The model under review builds one solid part; all positions refer to its coordinate system, in mm. Face numbers are marked on the shaded views. A direction names the side the tool comes from. Round coordinates to 2 decimals unless told otherwise and drop trailing zeros. Order: outer loops, then holes, each group sorted by start corner. A loop starts at its lowest first (then second) coordinate and runs counter-clockwise, first axis right, second up.
1) Machinability: for the marked faces 1 and 2, which of the approach directions +Z, -Z, +X, -X, +Y, -Y give a long, thin tool a straight path to every point of the face, cutting with its end or side? Answer none if there is none.
2) Consider section B-B (y = 5). Give the boundary of the cut face in (x, z) (3 decimals).
3) Mouldability with a two-part tool opening along Z and no side actions: class the marked faces 3 and 4 as pulls with the +Z half, pulls with the -Z half, needs draft (parallel to the pull), parting line crosses it, or undercut.
4) Consider section C-C (z = -12.5). Give the boundary of the cut face in (x, y), then the cut area to 3 significant figures.
5) Consider section A-A (z = -36). Give the boundary of the cut face in (x, y) (3 decimals), then the cut area to 3 significant figures.
6) Clearance check with flat-ended pins moving along their axes: P1, Ø0.6, axis at y = 0.5, z = -29.5, coming from the +X side (3 decimals); P2, Ø1.2, axis at x = 0, z = -36, coming from the +Y side; P3, Ø1.6, axis at y = 1, z = -8.5, coming from the +X side; P4, Ø2, axis at x = 26.5, y = 5, coming from the -Z side. State where each tip first meets the part, or that it passes through.
7) To check wall thickness, follow L1, parallel to X at y = 2.8, z = -7.5 (3 decimals); L2, parallel to Z at x = -12, y = 3.5; L3, parallel to X at y = 1.25, z = -6.5. State the ranges of each line that lie inside material, in increasing order.
from build123d import *

# Parameters (mm, degrees)
SALIENTE_EXTRUIR1_DEPTH = 4
SALIENTE_EXTRUIR2_START = 4
SALIENTE_EXTRUIR2_DEPTH = 4
REDONDEO1_R             = 10
REDONDEO3_R             = 2
CROQUIS3_R              = 1
CROQUIS3_R_2            = 9
CORTAR_EXTRUIR1_DEPTH   = 2
CROQUIS3_3_R            = 1
CORTAR_EXTRUIR2_DEPTH   = 77.740023923


with BuildPart() as part:
    # Croquis1 → Saliente-Extruir1 (new body)
    with BuildSketch(Plane(origin=(0, 0, 0), x_dir=(1, 0, 0), z_dir=(0, 1, 0))):
        with BuildLine():
            Line((30.125, 7.5), (25.125, 7.5))
            Line((25.125, 7.5), (25.125, 48))
            Line((25.125, 48), (30.125, 48))
            ThreePointArc((30.125, 48), (23.644737534, 63.644737534), (8, 70.125))
            Line((8, 70.125), (8, 65.125))
            Line((8, 65.125), (-8, 65.125))
            Line((-8, 65.125), (-8, 70.125))
            ThreePointArc((-8, 70.125), (-23.644737534, 63.644737534), (-30.125, 48))
            Line((-30.125, 48), (-25.125, 48))
            Line((-25.125, 48), (-25.125, 7.5))
            Line((-25.125, 7.5), (-30.125, 7.5))
            ThreePointArc((-30.125, 7.5), (-26.427223112, -1.427223112), (-17.5, -5.125))
            Line((-17.5, -5.125), (-17.5, -0.125))
            Line((-17.5, -0.125), (17.5, -0.125))
            Line((17.5, -0.125), (17.5, -5.125))
            ThreePointArc((17.5, -5.125), (26.427223112, -1.427223112), (30.125, 7.5))
        make_face()
    extrude(amount=SALIENTE_EXTRUIR1_DEPTH)

    # Croquis1<3> → Saliente-Extruir2 (add)
    with BuildSketch(Plane(origin=(0, 0, 0), x_dir=(1, 0, 0), z_dir=(0, 1, 0)).offset(SALIENTE_EXTRUIR2_START)):
        with BuildLine():
            Line((-30.125, 48), (-25.125, 48))
            ThreePointArc((-25.125, 48), (-20.109203628, 60.109203628), (-8, 65.125))
            Line((-8, 65.125), (-8, 70.125))
            ThreePointArc((-8, 70.125), (-23.644737534, 63.644737534), (-30.125, 48))
        make_face()
        with BuildLine():
            Line((-17.5, -5.125), (-17.5, -0.125))
            ThreePointArc((-17.5, -0.125), (-22.891689207, 2.108310793), (-25.125, 7.5))
            Line((-25.125, 7.5), (-30.125, 7.5))
            ThreePointArc((-30.125, 7.5), (-26.427223112, -1.427223112), (-17.5, -5.125))
        make_face()
        with BuildLine():
            ThreePointArc((25.125, 7.5), (22.891689207, 2.108310793), (17.5, -0.125))
            Line((17.5, -0.125), (17.5, -5.125))
            ThreePointArc((17.5, -5.125), (26.427223112, -1.427223112), (30.125, 7.5))
            Line((30.125, 7.5), (25.125, 7.5))
        make_face()
        with BuildLine():
            ThreePointArc((8, 65.125), (20.109203628, 60.109203628), (25.125, 48))
            Line((25.125, 48), (30.125, 48))
            ThreePointArc((30.125, 48), (23.644737534, 63.644737534), (8, 70.125))
            Line((8, 70.125), (8, 65.125))
        make_face()
    extrude(amount=SALIENTE_EXTRUIR2_DEPTH)

    # Redondeo1
    # the kernel refuses this fillet: 10 mm, written as the material it adds along each edge
    with BuildSketch(Plane(origin=(8, 0, -65.125), x_dir=(-1, 0, 0), z_dir=(0, 1, 0)), Plane(origin=(-17.5, 0, 0.125), x_dir=(1, 0, 0), z_dir=(0, 1, 0)), Plane(origin=(-25.125, 0, -48), x_dir=(0, 0, 1), z_dir=(0, 1, 0))) as redondeo1_piece_1:
        with BuildLine():
            CenterArc((8.660254038, -10), REDONDEO1_R, 90, 60)
            Line((0, -5), (-0.173205081, -4.9))
            ThreePointArc((-0.173205081, -4.9), (-0.2, -2.5), (-0.2, 0))
            Line((-0.2, 0), (0, 0.2))
            Line((0, 0.2), (8.660254038, 0.2))
            Line((8.660254038, 0.2), (8.660254038, 0))
        make_face()
    extrude(amount=4)
    with BuildSketch(Plane(origin=(-8, 0, -65.125), x_dir=(0, 0, -1), z_dir=(0, 1, 0)), Plane(origin=(17.5, 0, 0.125), x_dir=(0, 0, 1), z_dir=(0, 1, 0)), Plane(origin=(25.125, 0, -48), x_dir=(1, 0, 0), z_dir=(0, 1, 0)), Plane(origin=(-25.125, 0, -7.5), x_dir=(-1, 0, 0), z_dir=(0, 1, 0))) as redondeo1_piece_2:
        with BuildLine():
            CenterArc((10, -8.660254038), REDONDEO1_R, 120, 60)
            Line((0, -8.660254038), (-0.2, -8.660254038))
            Line((-0.2, -8.660254038), (-0.2, 0))
            Line((-0.2, 0), (0, 0.2))
            ThreePointArc((0, 0.2), (2.5, 0.2), (4.9, 0.173205081))
            Line((4.9, 0.173205081), (5, 0))
        make_face()
    extrude(amount=4)
    with BuildSketch(Plane(origin=(25.125, 0, -7.5), x_dir=(1, 0, 0), z_dir=(0, 1, 0))) as redondeo1_piece_3:
        with BuildLine():
            CenterArc((10, 8.660254038), REDONDEO1_R, 180, 60)
            Line((0, 8.660254038), (-0.2, 8.660254038))
            Line((-0.2, 8.660254038), (-0.2, 0))
            Line((-0.2, 0), (0, -0.2))
            ThreePointArc((0, -0.2), (2.5, -0.2), (4.9, -0.173205081))
            Line((4.9, -0.173205081), (5, 0))
        make_face()
    extrude(amount=4)

    # Redondeo3
    redondeo3_edges = [part.edges().sort_by_distance(p)[0] for p in [
        (-23.644737534, 8, -63.644737534),
        (-26.427223112, 8, 1.427223112),
        (26.427223112, 8, 1.427223112),
        (23.644737534, 8, -63.644737534),
    ]]
    fillet(redondeo3_edges, radius=REDONDEO3_R)

    # Croquis3 → Cortar-Extruir1 (cut)
    # profile 1 of 5: a face of its own
    with BuildSketch(Plane(origin=(0, 0, 0), x_dir=(1, 0, 0), z_dir=(0, 1, 0))):
        with BuildLine():
            ThreePointArc((-9.5, 10.354191767), (-3, 19), (-9.5, 27.645808233))
            Line((-9.5, 27.645808233), (-9.5, 31.845808233))
            ThreePointArc((-9.5, 31.845808233), (-10.144365081, 33.401443152), (-11.7, 34.045808233))
            Line((-11.7, 34.045808233), (-12.3, 34.045808233))
            ThreePointArc((-12.3, 34.045808233), (-13.855634919, 33.401443152), (-14.5, 31.845808233))
            Line((-14.5, 31.845808233), (-14.5, 27.645808233))
            ThreePointArc((-14.5, 27.645808233), (-21, 19), (-14.5, 10.354191767))
            Line((-14.5, 10.354191767), (-14.5, 6.154191767))
            ThreePointArc((-14.5, 6.154191767), (-13.855634919, 4.598556848), (-12.3, 3.954191767))
            Line((-12.3, 3.954191767), (-11.7, 3.954191767))
            ThreePointArc((-11.7, 3.954191767), (-10.144365081, 4.598556848), (-9.5, 6.154191767))
            Line((-9.5, 6.154191767), (-9.5, 10.354191767))
        make_face()
        with Locations(Location((-12, 7.5, 0), (0, 0, 90))):
            Circle(CROQUIS3_R, mode=Mode.SUBTRACT)
        with Locations(Location((-12, 30.5, 0), (0, 0, 90))):
            Circle(CROQUIS3_R, mode=Mode.SUBTRACT)
    # profile 2 of 5: a face of its own
    with BuildSketch(Plane(origin=(0, 0, 0), x_dir=(1, 0, 0), z_dir=(0, 1, 0))):
        with BuildLine():
            Line((14.5, 27.645808233), (14.5, 31.845808233))
            ThreePointArc((14.5, 31.845808233), (13.855634919, 33.401443152), (12.3, 34.045808233))
            Line((12.3, 34.045808233), (11.7, 34.045808233))
            ThreePointArc((11.7, 34.045808233), (10.144365081, 33.401443152), (9.5, 31.845808233))
            Line((9.5, 31.845808233), (9.5, 27.645808233))
            ThreePointArc((9.5, 27.645808233), (3, 19), (9.5, 10.354191767))
            Line((9.5, 10.354191767), (9.5, 6.154191767))
            ThreePointArc((9.5, 6.154191767), (10.144365081, 4.598556848), (11.7, 3.954191767))
            Line((11.7, 3.954191767), (12.3, 3.954191767))
            ThreePointArc((12.3, 3.954191767), (13.855634919, 4.598556848), (14.5, 6.154191767))
            Line((14.5, 6.154191767), (14.5, 10.354191767))
            ThreePointArc((14.5, 10.354191767), (21, 19), (14.5, 27.645808233))
        make_face()
        with Locations(Location((12, 7.5, 0), (0, 0, 90))):
            Circle(CROQUIS3_R, mode=Mode.SUBTRACT)
        with Locations(Location((12, 30.5, 0), (0, 0, 90))):
            Circle(CROQUIS3_R, mode=Mode.SUBTRACT)
    # profile 3 of 5: a face of its own
    with BuildSketch(Plane(origin=(0, 0, 0), x_dir=(1, 0, 0), z_dir=(0, 1, 0))):
        with Locations((0, 47.5)):
            Circle(CROQUIS3_R_2)
    # profile 4 of 5: a face of its own
    with BuildSketch(Plane(origin=(0, 0, 0), x_dir=(1, 0, 0), z_dir=(0, 1, 0))):
        with BuildLine():
            Line((2.5, 34.654191767), (2.5, 38.854191767))
            ThreePointArc((2.5, 38.854191767), (0, 38.5), (-2.5, 38.854191767))
            Line((-2.5, 38.854191767), (-2.5, 34.654191767))
            ThreePointArc((-2.5, 34.654191767), (-1.855634919, 33.098556848), (-0.3, 32.454191767))
            Line((-0.3, 32.454191767), (0.3, 32.454191767))
            ThreePointArc((0.3, 32.454191767), (1.855634919, 33.098556848), (2.5, 34.654191767))
        make_face()
        with Locations(Location((0, 36, 0), (0, 0, 90))):
            Circle(CROQUIS3_R, mode=Mode.SUBTRACT)
    # profile 5 of 5: a face of its own
    with BuildSketch(Plane(origin=(0, 0, 0), x_dir=(1, 0, 0), z_dir=(0, 1, 0))):
        with BuildLine():
            ThreePointArc((-2.5, 56.145808233), (0, 56.5), (2.5, 56.145808233))
            Line((2.5, 56.145808233), (2.5, 60.345808233))
            ThreePointArc((2.5, 60.345808233), (1.855634919, 61.901443152), (0.3, 62.545808233))
            Line((0.3, 62.545808233), (-0.3, 62.545808233))
            ThreePointArc((-0.3, 62.545808233), (-1.855634919, 61.901443152), (-2.5, 60.345808233))
            Line((-2.5, 60.345808233), (-2.5, 56.145808233))
        make_face()
        with Locations(Location((0, 59, 0), (0, 0, 90))):
            Circle(CROQUIS3_R, mode=Mode.SUBTRACT)
    extrude(amount=CORTAR_EXTRUIR1_DEPTH, mode=Mode.SUBTRACT)

    # Croquis3<3> → Cortar-Extruir2 (cut, through all)
    with BuildSketch(Plane(origin=(0, 0, 0), x_dir=(1, 0, 0), z_dir=(0, 1, 0))):
        with Locations(Location((-12, 7.5, 0), (0, 0, 90))):
            Circle(CROQUIS3_3_R)
        with Locations(Location((-12, 30.5, 0), (0, 0, 90))):
            Circle(CROQUIS3_3_R)
        with Locations(Location((12, 7.5, 0), (0, 0, 90))):
            Circle(CROQUIS3_3_R)
        with Locations(Location((12, 30.5, 0), (0, 0, 90))):
            Circle(CROQUIS3_3_R)
        with Locations(Location((0, 59, 0), (0, 0, 90))):
            Circle(CROQUIS3_3_R)
        with Locations(Location((0, 36, 0), (0, 0, 90))):
            Circle(CROQUIS3_3_R)
    extrude(amount=CORTAR_EXTRUIR2_DEPTH, mode=Mode.SUBTRACT)


solid = part.part
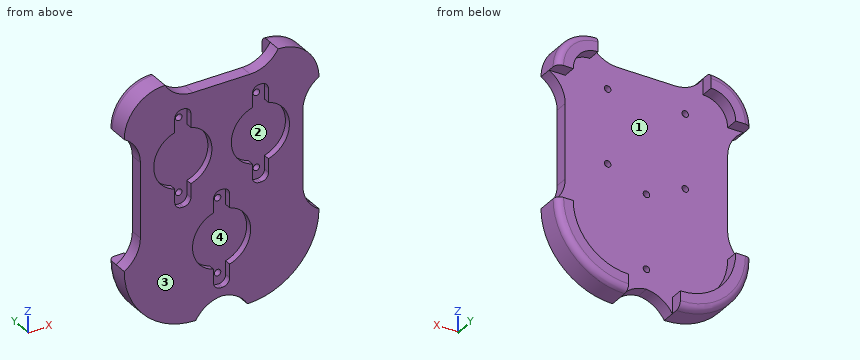
Answer below:
1. face 1: +Y
1. face 2: -Y
2. outline: (-30.125, -48) arc R22.125 ccw to (-8, -70.125) - (-8, -65.125) arc R17.125 cw to (-25.125, -48) - close; (-30.125, -7.5) - (-25.125, -7.5) arc R7.625 cw to (-17.5, 0.125) - (-17.5, 5.125) arc R12.625 ccw to start; (8, -70.125) arc R22.125 ccw to (30.125, -48) - (25.125, -48) arc R17.125 cw to (8, -65.125) - close; (17.5, 0.125) arc R7.625 cw to (25.125, -7.5) - (30.125, -7.5) arc R12.625 ccw to (17.5, 5.125) - close
3. face 3: needs draft
3. face 4: undercut
4. outline: (-25.82, 0) - (-18.22, 0) - (-18.22, 2) - (-5.78, 2) - (-5.78, 0) - (5.78, 0) - (5.78, 2) - (18.22, 2) - (18.22, 0) - (25.82, 0) - (25.82, 4) - (-25.82, 4) - close
4. area: 157 mm2
5. outline: (-25.125, 0) - (-2.5, 0) - (-2.5, 2) - (-1, 2) - (-1, 4) - (-25.125, 4) - close; (1, 2) - (2.5, 2) - (2.5, 0) - (25.125, 0) - (25.125, 4) - (1, 4) - close
5. area: 187 mm2
6. P1: stops at x = 25.125
6. P2: passes through
6. P3: stops at x = 29.79
6. P4: stops at z = -61.54
7. L1: x = -30.125 to -13, -11 to 11, 13 to 30.125
7. L2: z = -69.76 to -31.5, -29.5 to -8.5, -6.5 to 0.64
7. L3: x = -30.09 to -14.5, -9.5 to 9.5, 14.5 to 30.09
